Here's how the part is built. I have some questions about the finished solid (model axes, mm). A direction names the side the tool comes from. Round coordinates to 2 decimals unless told otherwise and drop trailing zeros. Order: outer loops, then holes, each group sorted by start corner. A loop starts at its lowest first (then second) coordinate and runs counter-clockwise, first axis right, second up.
```python
from build123d import *

# Parameters (mm, degrees)
PAD_DEPTH       = 12
POCKET_DEPTH    = 62
SKETCH019_W     = 31
SKETCH019_H     = 21.780884
POCKET002_DEPTH = 17
SKETCH020_R     = 2
POCKET003_DEPTH = 4


with BuildPart() as part:
    # Sketch010 → Pad (new body, symmetric)
    with BuildSketch(Plane.XY):
        with BuildLine():
            Line((12.639868, 59.984547), (-12.639868, 59.984547))
            Line((-12.639868, 59.984547), (-17.867889, 82.058411))
            Line((-17.867889, 82.058411), (-17.867889, 102.222236))
            ThreePointArc((-15.867889, 104.222236), (-17.282103, 103.63645), (-17.867889, 102.222236))
            Line((-15.867889, 104.222236), (-8.154342, 104.222236))
            ThreePointArc((-7.154342, 103.222236), (-7.447235, 103.929343), (-8.154342, 104.222236))
            Line((-7.154342, 103.222236), (-7.154342, 92.189331))
            Line((-7.154342, 92.189331), (7.154342, 92.189331))
            Line((7.154342, 92.189331), (7.154342, 103.222236))
            ThreePointArc((8.154342, 104.222236), (7.447235, 103.929343), (7.154342, 103.222236))
            Line((8.154342, 104.222236), (15.867889, 104.222236))
            ThreePointArc((17.867889, 102.222236), (17.282103, 103.63645), (15.867889, 104.222236))
            Line((17.867889, 102.222236), (17.867889, 82.058411))
            Line((17.867889, 82.058411), (12.639868, 59.984547))
        make_face()
    extrude(amount=PAD_DEPTH, both=True)

    # Sketch011 → Pocket (cut)
    with BuildSketch(Plane.XZ.offset(-54)):
        Polygon((0, 13.813917), (-22.117895, 13.813917), (-22.117895, -0.189388), (-22.117895, -17.743416), (0, -17.743416), (22.658901, -17.743416), (22.658901, -0.111897), (22.658901, 13.813917), align=None)
        Polygon((-18.596464, 0), (-18.596464, 5.287208), (-8.154342, 8), (-7.443202, 8.179805), (0, 8.179805), (7.519913, 8.179805), (8.154342, 8), (18.531284, 5.287208), (18.531284, -0.112287), (18.531284, -5.399495), (8.154342, -8), (7.554242, -8.253323), (0.11104, -8.253323), (-7.443202, -8.253323), (-8.154342, -8), (-18.596464, -5.371119), align=None, mode=Mode.SUBTRACT)
    extrude(amount=-POCKET_DEPTH, mode=Mode.SUBTRACT)

    # Sketch019 → Pocket002 (cut)
    with BuildSketch(Plane.XY.offset(0.8)):
        with Locations((0.01352, 95.005211)):
            Rectangle(SKETCH019_W, SKETCH019_H)
    extrude(amount=-POCKET002_DEPTH, mode=Mode.SUBTRACT)

    # Sketch020 → Pocket003 (cut)
    with BuildSketch(Plane.XY.offset(0.8)):
        with Locations((-11.1, 94.9)):
            Circle(SKETCH020_R)
        with Locations((11.3, 94.9)):
            Circle(SKETCH020_R)
        with Locations((0.013518, 88.3)):
            Circle(SKETCH020_R)
    extrude(amount=POCKET003_DEPTH, mode=Mode.SUBTRACT)


solid = part.part
```
1) I'm going to push flat-ended pins straight in: pin 1 (2 mm diameter, centred on x = 0.5, y = 89, fed in from -Z); pin 2 (3 mm diameter, centred on x = 2.5, z = 5, fed in from +Y); pin 3 (4.5 mm diameter, centred on x = -10.5, y = 94, fed in from -Z). Where does each tip first touch, or does it pass through?
2) If we section it at B-B (z = -0.75): Write out the boundary of the cut face in (x, y).
3) If we section it at D-D (y = 100.5): Write out the boundary of the cut face in (x, z).
4) If we section it at C-C (z = 3.25): Write out the boundary of the cut face in (x, y).
5) For faces 4 (the flat face through (0, 84.115, -4)), 5 (the cylindrical face through (-0.42, 86.348, 2.772)), 6 (the cylindrical face through (7.46, 103.94, 4.54)), which set-ups out of +Z, -Z, +X, -X, +Y, -Y let a thin tool reach every point of the face, with its end or its side?
6) If we section it at A-A (y = 94.9): Write out the boundary of the cut face in (x, z).
7) We'd pull the mould along Y, two halves only. Please class faces 1 (the flat face through (15.29, 71.18, 0.07)), 2 (the cylindrical face through (10.866, 92.948, 2.772)), 3 (the flat face through (-12.943, 76.878, -6.794)): +Y half, -Y half, draft (parallel to the pull), parting line (faces both ways), or undercut.
8) I need wall thicknesses on line 1 (X direction, y = 93.5, z = -5); line 2 (Y direction, x = -11.1, z = 2.1); line 3 (Y direction, x = 2.5, z = -5). Which ranges of each line are inside material? Lowest first, please.
Solutions:
1. pin 1: stops at z = 4.8
1. pin 2: stops at y = 92.19
1. pin 3: stops at z = 0.8
2. outline: (-17.87, 82.06) - (-12.64, 59.98) - (12.64, 59.98) - (17.87, 82.06) - (17.87, 102.22) arc R2 ccw to (15.87, 104.22) - (15.51, 104.22) - (15.51, 84.11) - (-15.49, 84.11) - (-15.49, 104.22) - (-15.87, 104.22) arc R2 ccw to (-17.87, 102.22) - close
3. outline: (-17.87, -5.55) - (-15.49, -6.15) - (-15.49, 0.8) - (-7.15, 0.8) - (-7.15, 8.18) - (-7.44, 8.18) - (-8.15, 8) - (-17.87, 5.48) - close; (7.15, 0.8) - (15.51, 0.8) - (15.51, -6.16) - (17.87, -5.57) - (17.87, 5.46) - (8.15, 8) - (7.52, 8.18) - (7.15, 8.18) - close
4. outline: (-17.87, 82.06) - (-12.64, 59.98) - (12.64, 59.98) - (17.87, 82.06) - (17.87, 102.22) arc R2 ccw to (15.87, 104.22) - (8.15, 104.22) arc R1 ccw to (7.15, 103.22) - (7.15, 92.19) - (-7.15, 92.19) - (-7.15, 103.22) arc R1 ccw to (-8.15, 104.22) - (-15.87, 104.22) arc R2 ccw to (-17.87, 102.22) - close; hole circle Ø4 at (-11.1, 94.9); hole circle Ø4 at (0.01, 88.3); hole circle Ø4 at (11.3, 94.9)
5. face 4: -Z, +Y
5. face 5: -Z
5. face 6: +Z, -Z, +Y
6. outline: (-17.87, -5.55) - (-15.49, -6.15) - (-15.49, 0.8) - (-13.1, 0.8) - (-13.1, 4.8) - (-9.1, 4.8) - (-9.1, 0.8) - (-7.15, 0.8) - (-7.15, 8.18) - (-7.44, 8.18) - (-8.15, 8) - (-17.87, 5.48) - close; (7.15, 0.8) - (9.3, 0.8) - (9.3, 4.8) - (13.3, 4.8) - (13.3, 0.8) - (15.51, 0.8) - (15.51, -6.16) - (17.87, -5.57) - (17.87, 5.46) - (8.15, 8) - (7.52, 8.18) - (7.15, 8.18) - close
7. face 1: -Y half
7. face 2: undercut
7. face 3: draft
8. line 1: x = -17.87 to -15.49, 15.51 to 17.87
8. line 2: y = 59.98 to 92.9, 96.9 to 104.22
8. line 3: y = 59.98 to 84.11
